Design review of the part shown in the three views and the two pictorial views. Dimensions are in mm from the part's minimum x, y and z. Coordinates: 2 decimals unless noted, no trailing zeros. Write each loop counter-clockwise with the first axis right and the second up, starting at its lowest first coordinate (ties: lowest second). Pieces come first, ordered by that corner, then holes. Notation, with made-up numbers: (74, 52) -> (107, 52) arc R16 cw to (107, 62) -> close; hole circle Ø3 at (14, 1.5). An arc over 180 degrees is marked (long way). Write each question's results on one line, items separated by ' | '.
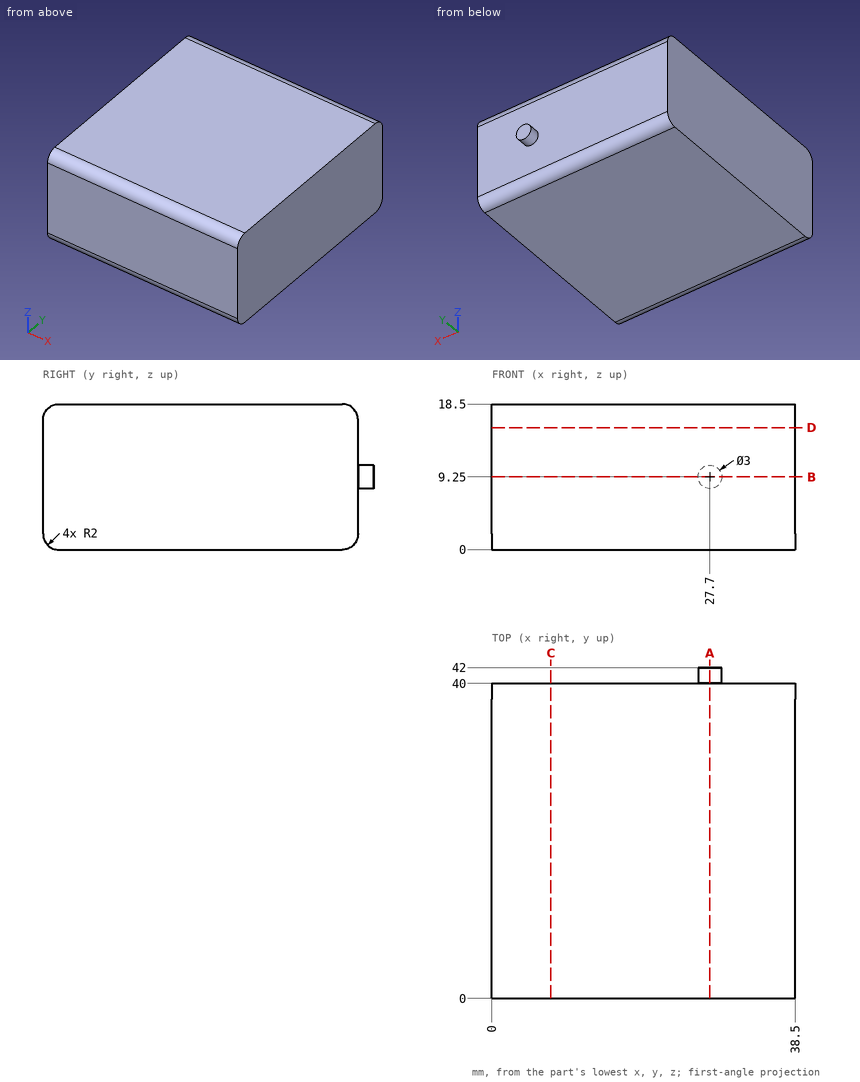
Q1. For line 1 (Y direction, x = 33.5, z = 3.5); line 2 (Y direction, x = 12.5, z = 17.5); line 3 (Z direction, x = 29, y = 40.5), list the stretches that pass through material, from the lowest coordinate up. Write a range as from..to.
Solution:
line 1: 0..40 | line 2: 0.27..39.73 | line 3: 8.5..10
Q2. Add section B-B (z = 9.25). Write out the cut boundary in (x, y), plus the area to 3 significant figures.
Solution:
outline: (0, 0) -> (38.5, 0) -> (38.5, 40) -> (29.2, 40) -> (29.2, 42) -> (26.2, 42) -> (26.2, 40) -> (0, 40) -> close | area: 1,550 mm²
Q3. Clearance check with a flat-ended pin moving along its axis: P1, Ø5, axis at x = 16.5, z = 9.5, coming from the -Y side. State where the tip first meets the part, or that it passes through.
Solution:
P1: y = 0
Q4. Add section D-D (z = 15.5). Write out the cut boundary in (x, y), plus the area to 3 significant figures.
Solution:
outline: (0, 0) -> (38.5, 0) -> (38.5, 40) -> (0, 40) -> close | area: 1,540 mm²
Q5. Add section A-A (x = 27.7). Write out the cut boundary in (y, z).
Solution:
outline: (0, 2) arc R2 ccw to (2, 0) -> (38, 0) arc R2 ccw to (40, 2) -> (40, 7.75) -> (42, 7.75) -> (42, 10.75) -> (40, 10.75) -> (40, 16.5) arc R2 ccw to (38, 18.5) -> (2, 18.5) arc R2 ccw to (0, 16.5) -> close
Q6. Add section C-C (x = 7.5). Write out the cut boundary in (y, z).
Solution:
outline: (0, 2) arc R2 ccw to (2, 0) -> (38, 0) arc R2 ccw to (40, 2) -> (40, 16.5) arc R2 ccw to (38, 18.5) -> (2, 18.5) arc R2 ccw to (0, 16.5) -> close
